Autodesk Inventor part; units mm, degrees
ref_plane "YZ Plane" through (0, 0, 0) normal (1, 0, 0) x (0, 1, 0)
ref_plane "XZ Plane" through (0, 0, 0) normal (0, 1, 0) x (-1, 0, 0)
ref_plane "XY Plane" through (0, 0, 0) normal (0, 0, 1) x (1, 0, 0)
sketch "Sketch1" plane through (0, 0, 0) normal (0, 1, 0) x (-1, 0, 0)
  circle A0 centre (0, 0) radius 1.5
  dimension "d0" = 3
extrude "Extrusion1" add sketch "Sketch1" along normal blind 116
sketch "Sketch2" plane through (0, 116, 0) normal (0, 1, 0) x (1, 0, 0)
  circle A0 centre (0, 0) radius 1.4
  dimension "d3" = 2.8
extrude "Extrusion2" add sketch "Sketch2" along normal blind 1
sketch "Sketch3" plane through (0, 117, 0) normal (0, 1, 0) x (1, 0, 0)
  circle A0 centre (0, 0) radius 1.5
  dimension "d6" = 3
extrude "Extrusion3" add sketch "Sketch3" along normal blind 10
thread "Thread1"
chamfer "Chamfer1" distance 0.3 angle 45 1 edges at (-1.5, 127, 0)
chamfer "Chamfer2" distance 0.3 angle 45 1 edges at (1.5, 0, 0)
sketch "Sketch4" plane through (0, 0, 0) normal (1, 0, 0) x (0, 1, 0)
  line L0 (117, -1.5) -> (117, 1.5)
  line L1 (126.7, -1.5) -> (126.7, 1.5)
  line L2 (126.7, -1.5) -> (126.7, 1.5)
  line L3 (127, 1.2) -> (127, -1.2)
  line L4 (128.5, 0.5) -> (125.5, 0.5)
  line L5 (125.5, 0.5) -> (125.5, -0.5)
  line L6 (125.5, -0.5) -> (128.5, -0.5)
  line L7 (128.5, -0.5) -> (128.5, 0.5)
  line L8 (127, 1.2) -> (127, -1.2)
  line L9 (128.5, 0.5) -> (125.5, -0.5) construction
  line L10 (125.5, 0.5) -> (128.5, -0.5) construction
  point P0 (0, 0)
  point P1 (127, 0)
  dimension "d17" = 3
  dimension "d18" = 1
extrude "Extrusion4" cut sketch "Sketch4" along normal mid plane 10
properties part number "wał_prowadzący_hamulca_długi" material "Aluminum 6061"
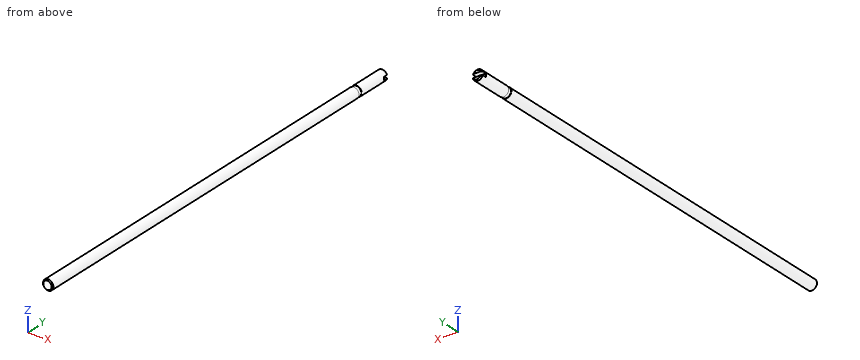
Read the model definition and answer for the solid it produces. Units are mm, in the model's axes. Give positions to 0.01 mm unless a question says otherwise; leave off trailing zeros. Write each loop counter-clockwise with the first axis right and the second up, starting at its lowest first coordinate (ties: lowest second). Pieces come first, ordered by that corner, then holes. Notation, with made-up numbers: (-36.75, 67) - (16.25, 67) arc R19 ccw to (16.25, 75) - close; hole circle Ø8 at (0, 23). An arc over 180 degrees is marked (long way). Return JSON: item names as keys, results as strings.
Q1. Given P1, Ø0.8, axis at x = 0.5, z = 0, coming from the +Y side, flat-ended and moving along its own axis, determine where the tip first touches the part or whether it passes through.
Reply:
{"P1": "y = 125.5"}
Q2. A cutting plane is placed at A-A, the plane y = 57. Determine the outline of the cut face in (x, z).
Reply:
{"outline": "circle Ø3 at (0, 0)"}
Q3. Consider line 1 along Y through (x, z) = (0.1, 0.45); line 2 along Z through (x, y) = (0.25, 77); line 3 along Z through (x, y) = (-0.5, 97). Determine where each line is inside the solid, lowest interval first. Write a range as [from, to].
Reply:
{"line 1": "[0, 125.5]", "line 2": "[-1.48, 1.48]", "line 3": "[-1.41, 1.41]"}
